from build123d import *

# Parameters (mm, degrees)
SKETCH2_R           = 19.5
CUT_EXTRUDE1_DEPTH  = 90
BOSS_EXTRUDE1_REACH = 112.853
SKETCH5_R           = 5
SKETCH6_R           = 1.5
CUT_EXTRUDE3_DEPTH  = 28


with BuildPart() as part:
    # Sketch1 → Revolve2 (revolve)
    with BuildSketch(Plane.XY):
        Polygon((0, 0), (25, 0), (25, -5.236486486), (44, -5.236486486), (44, -7.236486486), (62, -7.236486486), (62, -16.236486486), (30.5, -16.236486486), (30.5, -19.236486486), (26, -19.236486486), (26, -38.006756757), (0, -38.006756757), align=None)
    revolve(axis=Axis((0, -38.006756757, 0), (0, 1, 0)))

    # Sketch2 → Cut-Extrude1 (cut)
    with BuildSketch(Plane(origin=(0, 0, 0), x_dir=(1, 0, 0), z_dir=(0, 1, 0))):
        Circle(SKETCH2_R)
    extrude(amount=-CUT_EXTRUDE1_DEPTH, mode=Mode.SUBTRACT)

    # Boss-Extrude1: up to this face of the body (flat: up to its plane)
    boss_extrude1_end = Plane(part.part.faces().sort_by_distance((-45.753624817, -7.236486486, 0))[0])
    # Sketch5 → Boss-Extrude1 (add, up to the picked face)
    with BuildSketch(Plane(origin=(0, -1.236486486, -58), x_dir=(-1, 0, 0), z_dir=(0, 0.707106781, -0.707106781)), mode=Mode.PRIVATE) as boss_extrude1_sk1:
        Circle(SKETCH5_R)
    boss_extrude1_tool1 = split(extrude(boss_extrude1_sk1.sketch, amount=-BOSS_EXTRUDE1_REACH, mode=Mode.PRIVATE), bisect_by=boss_extrude1_end, keep=Keep.BOTH, mode=Mode.PRIVATE)
    add(boss_extrude1_tool1.solids().sort_by_distance((0, -1.236486, -58))[0])

    # Sketch6 → Cut-Extrude3 (cut)
    with BuildSketch(Plane(origin=(0, 28.381756757, -28.381756757), x_dir=(1, 0, 0), z_dir=(0, 0.707106781, -0.707106781))):
        with Locations((0, 41.886521288)):
            Circle(SKETCH6_R)
    extrude(amount=-CUT_EXTRUDE3_DEPTH, mode=Mode.SUBTRACT)


solid = part.part
Check sheet for the modelled part. Datum: model origin and axes. Units: mm. A direction names the side the tool comes from. Give positions to 0.01 mm unless a question says otherwise; leave off trailing zeros. Write each loop counter-clockwise with the first axis right and the second up, starting at its lowest first coordinate (ties: lowest second). Pieces come first, ordered by that corner, then holes. Notation, with made-up numbers: (22, 1) -> (71, 1) arc R22 cw to (71, 9) -> close; hole circle Ø7 at (78.25, -9). An arc over 180 degrees is marked (long way). Write item = value, one per line.
Item 1: Tool access check on faces 4 (the cylindrical face through (-9.538, -6.25, 42.954)), 5 (the flat face through (-15, 0, 13)), 6 (the cylindrical face through (-20.633, -28.753, 15.821)). Record the directions out of +Z, -Z, +X, -X, +Y, -Y that give a thin tool (end or side, any length) a straight path to the whole face; none if there is none.
Output:
face_4 = +Y
face_5 = +Z, +X, -X, +Y
face_6 = -Y
Item 2: Sectioned sample at C-C on y = -21. Record the boundary of the cut face in (x, z).
Output:
outline = circle Ø52 at (0, 0); hole circle Ø39 at (0, 0)
Item 3: Sectioned sample at D-D on z = 38.5. Record the boundary of the cut face in (x, y).
Output:
outline = (-48.6, -16.24) -> (48.6, -16.24) -> (48.6, -7.24) -> (21.3, -7.24) -> (21.3, -5.24) -> (-21.3, -5.24) -> (-21.3, -7.24) -> (-48.6, -7.24) -> close
Item 4: Release check for a two-part mould opening along Z. For faces 1 (the cylindrical face through (0.651, -1.373, -50.853)), 2 (the cylindrical face through (-8.071, -11.799, -61.472)), 3 (the flat face through (3.7, -38.007, -19.4)) record: +Z half, -Z half, draft (parallel to the pull), parting line (faces both ways), or undercut.
Output:
face_1 = undercut
face_2 = parting line
face_3 = draft
Item 5: Scan lines: probe 1 along X at (y, z) = (-23.5, 0); probe 2 along Z at (x, y) = (0, -11); probe 3 along X at (y, z) = (-9, 0). Record each from-to range of solid material in increasing order. Write a range as from..to.
Output:
probe_1 = -26..-19.5, 19.5..26
probe_2 = -62..-50.36, -46.12..-19.5, 19.5..62
probe_3 = -62..-19.5, 19.5..62
Item 6: Gauge pin test, flat ends, axial feed: pin 1 (1.5 mm diameter, centred on x = -21.5, y = -32.5, fed in from +Z); pin 2 (12 mm diameter, centred on y = -15.5, z = 32, fed in from -X) (3 decimals); pin 3 (4 mm diameter, centred on x = 32, z = -43.5, fed in from +Y). Record the tip position at first contact, or that the pin passes through.
Output:
pin_1 = 15.67
pin_2 = -56.285
pin_3 = -7.24
Item 7: Sectioned sample at B-B on x = 0. Count the separate pieces of the cut face and the enclosed holes in it, and give its area (3 significant figures).
Output:
separate_pieces = 3
enclosed_holes = 0
area = 1,250 mm^2
Item 8: Sectioned sample at A-A on z = 0. Record the boundary of the cut face in (x, y), and give its area (3 significant figures).
Output:
outline = (-62, -16.24) -> (-30.5, -16.24) -> (-30.5, -19.24) -> (-26, -19.24) -> (-26, -38.01) -> (-19.5, -38.01) -> (-19.5, 0) -> (-25, 0) -> (-25, -5.24) -> (-44, -5.24) -> (-44, -7.24) -> (-62, -7.24) -> close; (19.5, -38.01) -> (26, -38.01) -> (26, -19.24) -> (30.5, -19.24) -> (30.5, -16.24) -> (62, -16.24) -> (62, -7.24) -> (44, -7.24) -> (44, -5.24) -> (25, -5.24) -> (25, 0) -> (19.5, 0) -> close
area = 1,230 mm^2
